The listing builds one solid part. Answer for the finished solid, in the listing's coordinates (mm). Face numbers are marked on the shaded views. A direction names the side the tool comes from. Give positions to 0.01 mm unless a question says otherwise; leave off trailing zeros. Order: outer loops, then holes, each group sorted by start corner. A loop starts at its lowest first (then second) coordinate and runs counter-clockwise, first axis right, second up. Notation, with made-up numbers: (35, 16) - (50, 16) arc R7 cw to (50, 26) - close; hole circle Ø6 at (-37.5, 15). An arc over 180 degrees is marked (long way). Use a Markdown table: item, result. Add a question column.
1) The mould has two halves that part along X. Classify the marked faces 3, 4 and 5: released by +X, released by -X, zero draft, split by the parting line, or undercut.
2) Straight lines are drawn through the part: line 1 (Y direction, x = -47.5, z = -6.5); line 2 (X direction, y = 2, z = -8.5); line 3 (Y direction, x = -29, z = -16.25). For each, find the intervals that lie inside material, in ascending order.
3) Find section C-C, the plane x = -9. Determine the outline of the cut face in (y, z), plus the area to 3 significant figures.
4) Find section A-A, the plane y = -7.5. Determine the outline of the cut face in (x, z).
5) Flat-ended cylindrical pins translate along their axes: pin 1 (12 mm diameter, centred on y = 7, z = -19.5, fed in from +X); pin 2 (4 mm diameter, centred on x = -21, z = -18, fed in from +Y); pin 3 (1.5 mm diameter, centred on y = -7.5, z = -3, fed in from +X); pin 4 (6 mm diameter, centred on x = -29.5, z = -2.5, fed in from -Y). Find the tip coordinate at first contact, or state that the pin passes through.
6) For the marked faces 1 and 2, determine the directions among +Z, -Z, +X, -X, +Y, -Y from which every point of the face is accessible in a straight line to the end or side of a thin tool.
from build123d import *

# Parameters (mm, degrees)
REVOLUCI_N1_ANGLE     = 180
CROQUIS2_W            = 2
CROQUIS2_H            = 3
CORTAR_EXTRUIR1_DEPTH = 15
CROQUIS3_W            = 7.076217781
CROQUIS3_H            = 3
CROQUIS3_W_2          = 6.688868885
CORTAR_EXTRUIR2_DEPTH = 6.500003


with BuildPart() as part:
    # Croquis1 → Revolución1 (revolve)
    with BuildSketch(Plane.XY):
        with BuildLine():
            Line((-51.782166939, -4.382597623), (-31.532166939, -4.382597623))
            Line((-31.532166939, -4.382597623), (-31.532166939, -14.382597623))
            Line((-31.532166939, -14.382597623), (-31.532166939, -19.382597623))
            Line((-31.532166939, -19.382597623), (-36.748543174, -13.37211471))
            Line((-36.748543174, -13.37211471), (-36.748543174, -5.882597623))
            Line((-36.748543174, -5.882597623), (-43.248543174, -5.882597623))
            Line((-43.248543174, -5.882597623), (-53.282166939, -5.882597623))
            Line((-53.282166939, -5.882597623), (-53.282166939, -4.382597623))
            ThreePointArc((-53.282166939, -4.382597623), (-46.252729688, 12.587965125), (-29.282166939, 19.617402377))
            Line((-29.282166939, 19.617402377), (-29.282166939, 18.117402377))
            ThreePointArc((-29.282166939, 18.117402377), (-45.192069516, 11.527304954), (-51.782166939, -4.382597623))
        make_face()
    revolve(axis=Axis((-29.282166939, 19.617402377, 0), (0, -1, 0)), revolution_arc=REVOLUCI_N1_ANGLE)

    # Croquis2 → Cortar-Extruir1 (cut)
    with BuildSketch(Plane.XY):
        with Locations((-33.532166939, -7.382597623)):
            Rectangle(CROQUIS2_W, CROQUIS2_H)
        with Locations((-25.032166939, -7.382597623)):
            Rectangle(CROQUIS2_W, CROQUIS2_H)
        with Locations((-25.032166939, -11.382597623)):
            Rectangle(CROQUIS2_W, CROQUIS2_H)
        with Locations((-33.532166939, -11.382597623)):
            Rectangle(CROQUIS2_W, CROQUIS2_H)
    extrude(amount=-CORTAR_EXTRUIR1_DEPTH, mode=Mode.SUBTRACT)

    # Croquis3 → Cortar-Extruir2 (cut)
    with BuildSketch(Plane(origin=(-26.032166939, 0, 0), x_dir=(0, 0, -1), z_dir=(1, 0, 0))):
        with Locations((8.321249271, -11.382597623)):
            Rectangle(CROQUIS3_W, CROQUIS3_H)
        with Locations((8.127574822, -7.382597623)):
            Rectangle(CROQUIS3_W_2, CROQUIS3_H)
    extrude(amount=-CORTAR_EXTRUIR2_DEPTH, mode=Mode.SUBTRACT)


solid = part.part
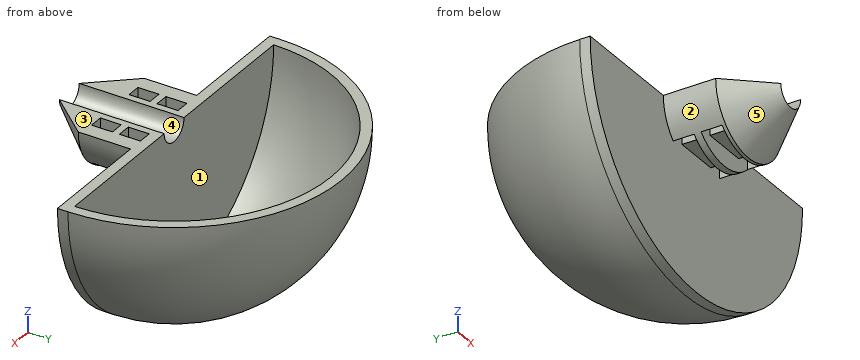
The answers:
| question | item | result |
|---|---|---|
| 1 | face 3 | zero draft |
| 1 | face 4 | undercut |
| 1 | face 5 | split by the parting line |
| 2 | line 1 | -5.88 to -4.38, 7.11 to 9.83 |
| 2 | line 2 | -50.8 to -49.11, -9.45 to -7.76 |
| 2 | line 3 | -5.88 to -4.38, 11.18 to 13.28 |
| 3 | outline | (-5.88, -12.83) - (-4.38, -12.83) arc R12.83 ccw to (8.45, 0) - (5.36, 0) arc R9.74 cw to (-4.38, -9.74) - (-4.38, 0) - (-5.88, 0) - close |
| 3 | area | 74.0 mm2 |
| 4 | outline | (-36.75, 0) arc R7.47 ccw to (-34.53, -5.31) - (-34.53, 0) - close; (-32.53, -4.78) - (-26.03, -4.78) - (-26.03, 0) - (-27.03, 0) arc R2.25 cw to (-31.53, 0) - (-32.53, 0) - close; (-24.03, -5.31) arc R7.47 ccw to (-21.82, 0) - (-24.03, 0) - close |
| 5 | pin 1 | x = -11.93 |
| 5 | pin 2 | y = 11.7 |
| 5 | pin 3 | x = -22.16 |
| 5 | pin 4 | y = -19.38 |
| 6 | face 1 | +Z |
| 6 | face 2 | -Z, -Y |
